```python
from build123d import *

# Parameters (mm, degrees)
EXTRUDE_1_DEPTH     = 9
EXTRUDE_2_DEPTH     = 5
SKETCH_3_R          = 6
CUT_EXTRUDE_1_DEPTH = 30
FILLET_1_R          = 2
EXTRUDE_3_DEPTH     = 5
EXTRUDE_5_DEPTH     = 2.5


with BuildPart() as part:
    # Sketch 1 → Extrude 1 (new, symmetric)
    with BuildSketch(Plane(origin=(0, 0, 0), x_dir=(0, 0, -1), z_dir=(1, 0, 0))):
        Polygon((-19.068057482, 16), (0, 0), (8.082464074, 0), (20.931942518, 0), (20.931942518, 20), (8.082464074, 20), (-19.068057482, 20), align=None)
    extrude(amount=EXTRUDE_1_DEPTH, both=True)

    # Sketch 1_3 → Extrude 2 (add, symmetric)
    with BuildSketch(Plane(origin=(0, 0, 0), x_dir=(0, 0, -1), z_dir=(1, 0, 0))):
        Polygon((20.931942518, 20), (20.931942518, 0), (45.931942518, 9.099255857), (45.931942518, 20), (30, 20), align=None)
        Polygon((40.931942518, 12.600293548), (25.931942518, 7.140740034), (25.931942518, 15), (40.931942518, 15), align=None, mode=Mode.SUBTRACT)
    extrude(amount=EXTRUDE_2_DEPTH, both=True)

    # Sketch 3 → Cut-Extrude 1 (cut)
    with BuildSketch(Plane(origin=(0, 20, 0), x_dir=(1, 0, 0), z_dir=(0, 1, 0))):
        with Locations(Location((0, -9, 0), (0, 0, 270))):
            Circle(SKETCH_3_R)
    extrude(amount=-CUT_EXTRUDE_1_DEPTH, mode=Mode.SUBTRACT)

    # Fillet 1
    fillet_1_edges = [part.edges().sort_by_distance(p)[0] for p in [
        (0, 16, 19.068057482),
        (0, 20, 19.068057482),
        (9, 18, 19.068057482),
        (-9, 18, 19.068057482),
    ]]
    fillet(fillet_1_edges, radius=FILLET_1_R)

    # Sketch 4 → Extrude 3 (add)
    with BuildSketch(Plane.XZ):
        Polygon((9, 0), (15, 0), (15, 4), (19, 4), (19, 0), (23, 0), (23, -4), (19, -4), (19, -8), (15, -8), (15, -4), (9, -4), align=None)
        Polygon((-23, 0), (-23, -4), (-19, -4), (-19, -8), (-15, -8), (-15, -4), (-9, -4), (-9, 0), (-15, 0), (-15, 4), (-19, 4), (-19, 0), align=None)
        Polygon((15, -16.931942518), (9, -16.931942518), (9, -20.931942518), (15, -20.931942518), (15, -24.931942518), (19, -24.931942518), (19, -20.931942518), (23, -20.931942518), (23, -16.931942518), (19, -16.931942518), (19, -12.931942518), (15, -12.931942518), align=None)
        Polygon((-19, -20.931942518), (-23, -20.931942518), (-23, -16.931942518), (-19, -16.931942518), (-19, -12.931942518), (-15, -12.931942518), (-15, -16.931942518), (-9, -16.931942518), (-9, -20.931942518), (-15, -20.931942518), (-15, -24.931942518), (-19, -24.931942518), align=None)
    extrude(amount=-EXTRUDE_3_DEPTH)

    # Sketch 5 → Extrude 5 (add, symmetric)
    with BuildSketch(Plane(origin=(0, 0, 0), x_dir=(0, 0, -1), z_dir=(1, 0, 0))):
        Polygon((0, 20), (0, 28), (15, 28), (15, 24), (20.931942518, 24), (20.931942518, 20), align=None)
    extrude(amount=EXTRUDE_5_DEPTH, both=True)


solid = part.part
```
Can you work these out from the model? Positions are in its coordinate system, mm. A direction names the side the tool comes from. Round coordinates to 2 decimals unless told otherwise and drop trailing zeros. Loops run counter-clockwise (first coordinate to the right, second up) from the corner with the lowest first, then second, coordinate; pieces in that order, holes last.
Item 1: Suppose I cut it at B-B, the plane z = 9. Write out the boundary of the cut face in (x, y).
Item 2: Suppose I cut it at D-D, the plane y = 6. Write out the boundary of the cut face in (x, z), then the cut area to 3 significant figures.
Item 3: Suppose I cut it at C-C, the plane x = -10. Write out the boundary of the cut face in (y, z), then the cut area to 3 significant figures.
Item 4: Please list where these lines run through material, in increasing order: L1, parallel to Z at x = 0, y = 13.25; L2, parallel to X at y = 14.5, z = 9; L3, parallel to Y at x = 3.5, z = -4.
Item 5: Suppose I cut it at A-A, the plane x = 0. Write out the boundary of the cut face in (y, z), then the cut area to 3 significant figures.
Item 6: Will these pins go through, and if not, where does the flat tip stop? pin 1 Ø9.5 at (x, z) = (-18, -19) entering from +Y; pin 2 Ø1.2 at (y, z) = (3.5, -24) entering from +X; pin 3 Ø5.5 at (x, y) = (12, 2) entering from +Z.
Item 7: Which directions (+Z, -Z, +X, -X, +Y, -Y) give clear straight access to the entire face, cutting with the end or side of a thin tool? Please do faces 4 (the flat face through (15, 2, -23)), 5 (the flat face through (-19, 2, -23)), 6 (the flat face through (-15, 2, -6)), 7 (the flat face through (21, 2, 0)).
Item 8: If we mould it in two halves opening along Z, with no side actions, what happens to faces 1 (the cylindrical face through (-8.65, 17.12, 18.2)), 2 (the flat face through (-19, 2, -15)), 3 (the flat face through (0, 24, -18))? For each: +Z half, -Z half, draft (parallel to the pull), parting line (faces both ways), or undercut.
Reported:
1. outline: (-9, 7.55) - (-6, 7.55) - (-6, 20) - (-9, 20) - close; (6, 7.55) - (9, 7.55) - (9, 20) - (6, 20) - close
2. outline: (-9, -20.93) - (-5, -20.93) - (-5, -37.42) - (5, -37.42) - (5, -20.93) - (9, -20.93) - (9, 7.15) - (5.71, 7.15) arc R6 cw to (-5.71, 7.15) - (-9, 7.15) - close
2. area: 636 mm2
3. outline: (0, -20.93) - (5, -20.93) - (5, -16.93) - (0, -16.93) - close; (0, -4) - (5, -4) - (5, 0) - (0, 0) - close
3. area: 40.0 mm2
4. L1: z = -45.93 to -40.93, -25.93 to 3, 15 to 15.79
4. L2: x = -9 to -6, 6 to 9
4. L3: y = 0 to 20
5. outline: (0, -20.93) - (9.1, -45.93) - (20, -45.93) - (20, -20.93) - (24, -20.93) - (24, -15) - (28, -15) - (28, 0) - (20, 0) - (20, 3) - (2.52, 3) - (0, 0) - close; (12.59, 15) - (20, 15) - (20, 17.07) arc R2 ccw to (18, 19.07) - (16.93, 19.07) arc R2 ccw to (15.4, 18.35) - close; hole (7.14, -25.93) - (12.6, -40.93) - (15, -40.93) - (15, -25.93) - close
5. area: 950 mm2
6. pin 1: stops at y = 5
6. pin 2: stops at x = 19
6. pin 3: stops at z = 0
7. face 4: -Z, +Y, -Y
7. face 5: -Z, -X, +Y, -Y
7. face 6: +Y, -Y
7. face 7: +Z, +X, +Y, -Y
8. face 1: +Z half
8. face 2: undercut
8. face 3: draft
